Can you work these out from the drawing? Everything is in mm from the part's minimum corner. A direction names the side the tool comes from. Round coordinates to 2 decimals unless told otherwise and drop trailing zeros. Loops run counter-clockwise (first coordinate to the right, second up) from the corner with the lowest first, then second, coordinate; pieces in that order, holes last. Notation, with made-up numbers: M 34.25,43.25 L 55.25,43.25 A26 ccw 55.25,75.25 Z; hole C -11.75,65.25 d1. An arc over 180 degrees is marked long. Answer in a Markdown table with one row per item.
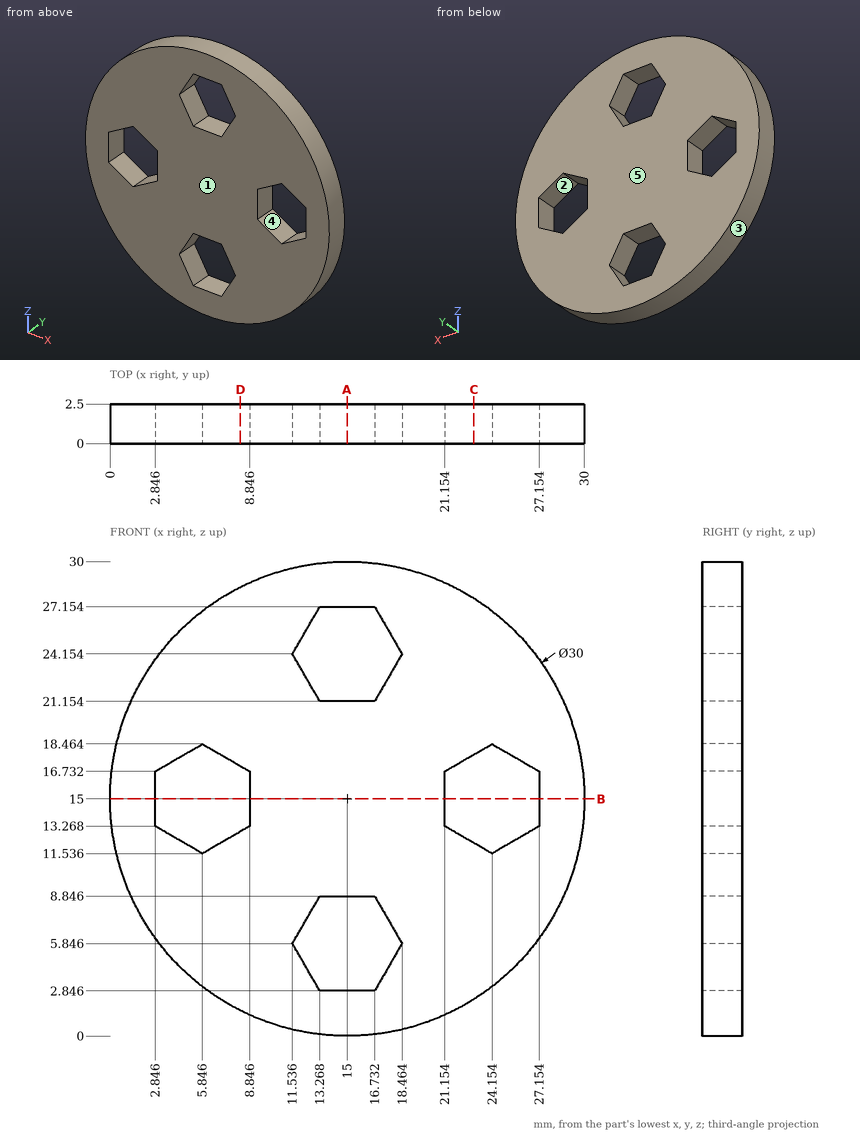
1) I want a section at D-D, the plane x = 8.25. Please give me the cut outline in (y, z).
Computed:
| item | result |
|---|---|
| outline | M 0,1.6 L 2.5,1.6 L 2.5,12.92 L 0,12.92 Z; M 0,17.08 L 2.5,17.08 L 2.5,28.4 L 0,28.4 Z |
2) I need wall thicknesses on line 1 (X direction, y = 1.65, z = 14.75); line 2 (Z direction, x = 17.75, y = 1.8) (1 decimal); line 3 (X direction, y = 2.35, z = 17.5) (1 decimal). Which ranges of each line are inside material? Lowest first, please.
Computed:
| item | result |
|---|---|
| line 1 | x = 0 to 2.85, 8.85 to 21.15, 27.15 to 30 |
| line 2 | z = 0.3 to 4.6, 7.1 to 22.9, 25.4 to 29.7 |
| line 3 | x = 0.2 to 4.2, 7.5 to 22.5, 25.8 to 29.8 |
3) I want a section at B-B, the plane z = 15. Please give me the cut outline in (x, y).
Computed:
| item | result |
|---|---|
| outline | M 0,0 L 2.85,0 L 2.85,2.5 L 0,2.5 Z; M 8.85,0 L 21.15,0 L 21.15,2.5 L 8.85,2.5 Z; M 27.15,0 L 30,0 L 30,2.5 L 27.15,2.5 Z |
4) I want a section at A-A, the plane x = 15. Please give me the cut outline in (y, z), plus the area to 3 significant figures.
Computed:
| item | result |
|---|---|
| outline | M 0,0 L 2.5,0 L 2.5,2.85 L 0,2.85 Z; M 0,8.85 L 2.5,8.85 L 2.5,21.15 L 0,21.15 Z; M 0,27.15 L 2.5,27.15 L 2.5,30 L 0,30 Z |
| area | 45.0 mm² |
5) Which directions (+Z, -Z, +X, -X, +Y, -Y) give clear straight access to the entire face, cutting with the end or side of a thin tool? Please do the marked faces 1 and 2.
Computed:
| item | result |
|---|---|
| face 1 | +Z, -Z, +X, -X, -Y |
| face 2 | +Y, -Y |
6) I want a section at C-C, the plane x = 23. Please give me the cut outline in (y, z).
Computed:
| item | result |
|---|---|
| outline | M 0,2.31 L 2.5,2.31 L 2.5,12.2 L 0,12.2 Z; M 0,17.8 L 2.5,17.8 L 2.5,27.69 L 0,27.69 Z |
7) If we mould it in two halves opening along Z, with no side actions, what happens to the marked faces 3, 4 and 5? For each: released by +Z, released by -Z, zero draft, split by the parting line, or undercut.
Computed:
| item | result |
|---|---|
| face 3 | split by the parting line |
| face 4 | undercut |
| face 5 | zero draft |
